Check sheet for the modelled part. Datum: model origin and axes. Units: mm. A direction names the side the tool comes from. Give positions to 0.01 mm unless a question says otherwise; leave off trailing zeros. Write each loop counter-clockwise with the first axis right and the second up, starting at its lowest first coordinate (ties: lowest second). Pieces come first, ordered by that corner, then holes. Notation, with made-up numbers: M -1.75,67.5 L 21.25,67.5 A26 cw 21.25,92.5 Z; hole C 32.5,-25 d4. An arc over 180 degrees is marked long. Write item = value, one per line. Start each with the question number.
1) Sectioned sample at A-A, the plane x = 0. Record the cut outline in (y, z).
2) Sectioned sample at C-C, the plane z = 0. Record the cut outline in (x, y).
3) Sectioned sample at B-B, the plane y = -1.3. Record the cut outline in (x, z), then the cut area to 3 significant figures.
4) Set-up check for faces 4 (the face through (0.759, -0.472, 3.417)), 5 (the face through (0, 1, -19)): record each of +Z, -Z, +X, -X, +Y, -Y from which the full face is reachable in a straight line by a thin tool's end or side.
5) Gauge pin test, flat ends, axial feed: pin 1 (3 mm diameter, centred on x = 2, z = -1, fed in from -Y); pin 2 (1 mm diameter, centred on y = -1.5, z = -15, fed in from +X); pin 3 (3.5 mm diameter, centred on x = 0, z = -14.5, fed in from -Y). Record the tip position at first contact, or that the pin passes through.
6) Scan lines: L1, parallel to Z at x = 0, y = -0.75; L2, parallel to Z at x = 0, y = 0.45; L3, parallel to Y at x = -0.25, z = -16. Record each from-to range of solid material in increasing order.
7) Sectioned sample at D-D, the plane y = 1.1. Record the cut outline in (x, z), then the cut area to 3 significant figures.
8) Draft check along Z on faces 1 (the face through (2.6, 0.99, -9.63)), 2 (the face through (0, 0, -10)), 3 (the face through (0.54, -0.99, -2.44)). Enter one of: pulls with the +Z half, pulls with the -Z half, needs draft (parallel to the pull), parting line crosses it, or undercut.
Autodesk Inventor part; units mm, degrees
ref_plane "YZ Plane" through (0, 0, 0) normal (1, 0, 0) x (0, 1, 0)
ref_plane "XZ Plane" through (0, 0, 0) normal (0, 1, 0) x (-1, 0, 0)
ref_plane "XY Plane" through (0, 0, 0) normal (0, 0, 1) x (1, 0, 0)
sketch "Sketch1" plane through (0, 0, 0) normal (0, 1, 0) x (-1, 0, 0)
  circle A0 centre (0, 0) radius 3.5
  line L0 (0, 3.5) -> (0, -18.5)
  circle A1 centre (0, -18.5) radius 1.75
  line L1 (1.7422, -18.6655) -> (3.4843, -0.3311)
  line L2 (-1.7422, -18.6655) -> (-3.4843, -0.3311)
  circle A2 centre (0, 0) radius 2.5
  circle A3 centre (0, -18.5) radius 0.5
  dimension "d0" = 7
  dimension "d1" = 22
  dimension "d2" = 3.5
  dimension "d3" = 5
  dimension "d8" = 1
extrude "Extrusion1" add sketch "Sketch1" along normal blind 2
extrude "Extrusion2" add sketch "Sketch1" against normal blind 2 contours A0 L0 A2 | L0 A2 A0
properties part number "servohorn" material "Acetal Resin, Black"
Data:
q1.outline = M -2,-3.5 L 0,-3.5 L 0,-18 L 2,-18 L 2,3.5 L -2,3.5 L -2,2.5 L 0,2.5 L 0,-2.5 L -2,-2.5 Z; M 0,-20.25 L 2,-20.25 L 2,-19 L 0,-19 Z
q2.outline = M -3.5,-2 L -2.5,-2 L -2.5,0 L 2.5,0 L 2.5,-2 L 3.5,-2 L 3.5,2 L -3.5,2 Z
q3.outline = C 0,0 d7; hole C 0,0 d5
q3.area = 18.8 mm2
q4.face_4 = -Y
q4.face_5 = +Y, -Y
q5.pin_1 = -2
q5.pin_2 = through
q5.pin_3 = 0
q6.L1 = -3.5 to -2.5, 2.5 to 3.5
q6.L2 = -20.25 to -19, -18 to 3.5
q6.L3 = 0 to 2
q7.outline = M -3.48,-0.33 L -1.74,-18.67 A1.75 ccw 1.74,-18.67 L 3.48,-0.33 A3.5 ccw long Z; hole C 0,-18.5 d1
q7.area = 121 mm2
q8.face_1 = pulls with the -Z half
q8.face_2 = needs draft
q8.face_3 = undercut
